Could you check a few things on this model? Use its own coordinates, in mm. Give positions to 0.01 mm unless a question says otherwise; leave off trailing zeros. Order: outer loops, then holes, each group sorted by start corner. A loop starts at its lowest first (then second) coordinate and runs counter-clockwise, first axis right, second up. Notation, with made-up numbers: (28, 52.25) -> (55, 52.25) arc R33 cw to (55, 85.25) -> close; hole circle Ø10 at (36, -13.5). An arc over 180 degrees is marked (long way). Write each question's results on one line, items separated by ' | '.
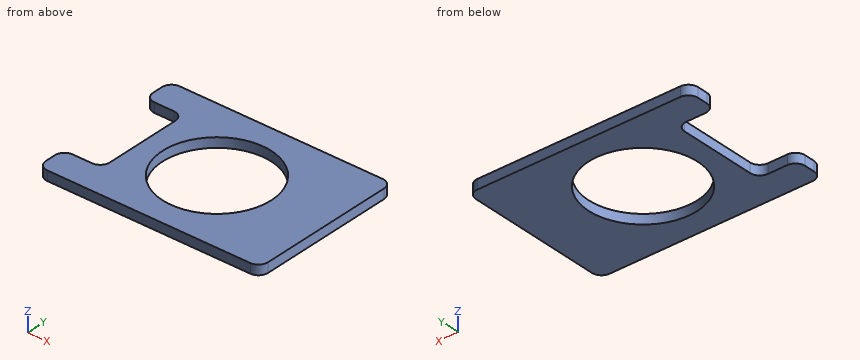
Autodesk Inventor part; units mm, degrees
ref_plane "YZ Plane" through (0, 0, 0) normal (1, 0, 0) x (0, 1, 0)
ref_plane "XZ Plane" through (0, 0, 0) normal (0, 1, 0) x (-1, 0, 0)
ref_plane "XY Plane" through (0, 0, 0) normal (0, 0, 1) x (1, 0, 0)
sketch "Sketch1" plane through (0, 0, 0) normal (0, 0, 1) x (1, 0, 0)
  line L0 (-23, -16.1697) -> (23, -16.1697)
  line L1 (23, -16.1697) -> (23, 16.1697)
  line L2 (23, 16.1697) -> (-23, 16.1697)
  line L3 (-23, 16.1697) -> (-23, -16.1697)
  line L4 (-23, -16.1697) -> (23, 16.1697) construction
  line L5 (23, -16.1697) -> (-23, 16.1697) construction
  line L6 (-32.2, 0) -> (32.2, 0)
  circle A0 centre (0.4, 0) radius 11.25
  point P0 (0, 0)
  dimension "d0" = 46
  dimension "d1" = 22.5
  dimension "d2" = 22.6
extrude "Extrusion1" add sketch "Sketch1" along normal blind 2 contours L3 L6 A0 L1 L0 | L3 L2 L1 L6 A0
sketch "Sketch2" plane through (0, 0, 2) normal (0, 0, 1) x (1, 0, 0)
  line L0 (-32.2, 0) -> (32.2, 0)
  line L1 (-15, -10) -> (-23, -10)
  line L2 (-23, -10) -> (-23, 10)
  line L3 (-23, 10) -> (-15, 10)
  line L4 (-15, 10) -> (-15, -10)
  line L5 (-15, -10) -> (-23, 10) construction
  line L6 (-23, -10) -> (-15, 10) construction
  line L7 (-23, 16.1697) -> (-23, -16.1697)
  point P0 (0, 0)
  point P1 (-19, 0)
  dimension "d5" = 20
  dimension "d8" = 8
extrude "Extrusion2" cut sketch "Sketch2" against normal through all
fillet "Fillet1" radius 2 8 edges at (-15, 10, 1) (-15, -10, 1) (-23, -10, 1) (-23, -16.1697, 1) (-23, 10, 1) (-23, 16.1697, 1) (23, -16.1697, 1) (23, 16.1697, 1)
properties part number "_3DPrint"
Q1. Suppose I cut it at A-A on z = 0.4. Please give me the cut outline in (x, y).
Here are the results:
outline: (-23, -14.17) arc R2 ccw to (-21, -16.17) -> (21, -16.17) arc R2 ccw to (23, -14.17) -> (23, 14.17) arc R2 ccw to (21, 16.17) -> (-21, 16.17) arc R2 ccw to (-23, 14.17) -> (-23, 12) arc R2 ccw to (-21, 10) -> (-17, 10) arc R2 cw to (-15, 8) -> (-15, -8) arc R2 cw to (-17, -10) -> (-21, -10) arc R2 ccw to (-23, -12) -> close; hole circle Ø22.5 at (0.4, 0)
Q2. Suppose I cut it at B-B on x = 0.4. Please give me the cut outline in (y, z), and give its area (3 significant figures).
Here are the results:
outline: (-16.17, 0) -> (-11.25, 0) -> (-11.25, 2) -> (-16.17, 2) -> close; (11.25, 0) -> (16.17, 0) -> (16.17, 2) -> (11.25, 2) -> close | area: 19.7 mm²
Q3. I'm going to push a flat-ended pin straight in: pin 1 Ø0.6 at (y, z) = (1, 1) entering from -X. Where does the tip first touch, or does it pass through?
Here are the results:
pin 1: stops at x = -15
Q4. I need wall thicknesses on line 1 along Y through (x, z) = (0.4, 1.6); line 2 along X through (y, z) = (0, 0.6); line 3 along Y through (x, z) = (-20.5, 0.1). Which ranges of each line are inside material? Lowest first, please.
Here are the results:
line 1: y = -16.17 to -11.25, 11.25 to 16.17 | line 2: x = -15 to -10.85, 11.65 to 23 | line 3: y = -16.17 to -10, 10 to 16.17
Q5. Suppose I cut it at C-C on y = 0. Please give me the cut outline in (x, z), and give its area (3 significant figures).
Here are the results:
outline: (-15, 0) -> (-10.85, 0) -> (-10.85, 2) -> (-15, 2) -> close; (11.65, 0) -> (23, 0) -> (23, 2) -> (11.65, 2) -> close | area: 31.0 mm²
